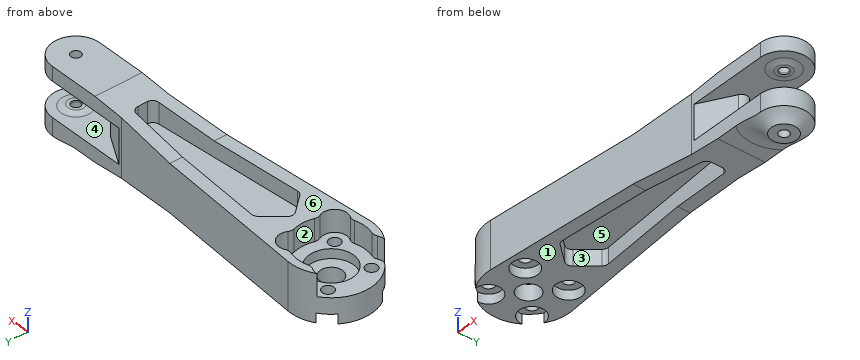
from build123d import *

# Parameters (mm, degrees)
SKETCH2_R               = 13
SKETCH2_R_2             = 7.5
BOSS_EXTRUDE2_DEPTH     = 10
CUT_EXTRUDE1_DEPTH      = 105.791459576
CUT_EXTRUDE1_DEPTH_BACK = 105.791459576
SKETCH5_R               = 1.83
SKETCH5_R_2             = 3.5
CUT_EXTRUDE2_DEPTH      = 106.770979007
HUB_CUTOUT_DEPTH        = 7
SKETCH8_R               = 7
CUT_EXTRUDE4_DEPTH      = 3
CUT_EXTRUDE5_DEPTH      = 105.791459576
CUT_EXTRUDE5_DEPTH_BACK = 105.791459576
SKETCH9_R               = 1.55
CUT_EXTRUDE6_DEPTH      = 5.5
FILLET1_R               = 2
CUT_EXTRUDE7_START      = 2.5
CUT_EXTRUDE7_DEPTH      = 103.291459576
FILLET2_R               = 2
FILLET2_OF_MIRROR1_R    = 2
SKETCH12_R              = 4
SKETCH12_R_2            = 1.55
BOSS_EXTRUDE3_DEPTH     = 4
FILLET3_START           = -14
FILLET3_2_DEPTH         = 4
BOSS_EXTRUDE4_START     = 5.5
SKETCH13_R              = 2.5
SKETCH13_R_2            = 1.5
BOSS_EXTRUDE4_DEPTH     = 0.5
BOSS_EXTRUDE5_START     = -5
SKETCH13_2_R            = 2.5
SKETCH13_2_R_2          = 1.5
BOSS_EXTRUDE5_DEPTH     = 0.5
FILLET4_R               = 5
SKETCH15_R              = 4
CUT_EXTRUDE8_DEPTH      = 3


with BuildPart() as part:
    # Sketch2 → Boss-Extrude2 (new, symmetric)
    with BuildSketch(Plane.XY):
        Circle(SKETCH2_R)
        with BuildLine():
            Line((70, 7.5), (1.025771359, 12.959467316))
            ThreePointArc((1.025771359, 12.959467316), (9.548168088, 8.822272166), (13, 0))
            ThreePointArc((13, 0), (9.548168088, -8.822272166), (1.025771359, -12.959467316))
            Line((1.025771359, -12.959467316), (70, -7.5))
            Line((70, -7.5), (70, 7.5))
        make_face()
        with BuildLine():
            Line((96, 7.5), (70, 7.5))
            Line((70, 7.5), (70, -7.5))
            Line((70, -7.5), (96, -7.5))
            ThreePointArc((96, -7.5), (88.5, 0), (96, 7.5))
        make_face()
        with Locations((96, 0)):
            Circle(SKETCH2_R_2)
        Circle(SKETCH2_R)
    extrude(amount=BOSS_EXTRUDE2_DEPTH, both=True)

    # Sketch4 → Cut-Extrude1 (cut, two sides: drawn at the far end of the back side and taken through both)
    with BuildSketch(Plane(origin=(0, 0, 0), x_dir=(1, 0, 0), z_dir=(0, 1, 0)).offset(-CUT_EXTRUDE1_DEPTH_BACK)):
        Polygon((-13, 7.5), (50, 7.5), (80, 10), (-13, 10), align=None)
        Polygon((-13, -7.5), (50, -7.5), (80, -10), (-13, -10), align=None)
    extrude(amount=CUT_EXTRUDE1_DEPTH + CUT_EXTRUDE1_DEPTH_BACK, mode=Mode.SUBTRACT)

    # Sketch5 → Cut-Extrude2 (cut, through all)
    with BuildSketch(Plane.XY.offset(7.5)):
        with Locations((-6.914797213, 6.914797213)):
            Circle(SKETCH5_R)
        with Locations((6.914797213, 6.914797213)):
            Circle(SKETCH5_R)
        with Locations((6.914797213, -6.914797213)):
            Circle(SKETCH5_R)
        with Locations((-6.914797213, -6.914797213)):
            Circle(SKETCH5_R)
        Circle(SKETCH5_R_2)
    extrude(amount=-CUT_EXTRUDE2_DEPTH, mode=Mode.SUBTRACT)

    # Sketch7 → hub cutout (cut)
    with BuildSketch(Plane.XY.offset(7.5)):
        with BuildLine():
            ThreePointArc((-7.281143007, 10.769631215), (-13, 0), (-7.281143007, -10.769631215))
            ThreePointArc((-7.281143007, -10.769631215), (-6.15529138, -10.711783559), (-5.093815501, -10.332103173))
            ThreePointArc((-5.093815501, -10.332103173), (-4.17580433, -10.057753531), (-3.223255475, -10.161014917))
            ThreePointArc((-3.223255475, -10.161014917), (0, -10.66), (3.223255475, -10.161014917))
            ThreePointArc((3.223255475, -10.161014917), (4.17580433, -10.057753531), (5.093815501, -10.332103173))
            ThreePointArc((5.093815501, -10.332103173), (9.652858062, -9.652858062), (10.332103173, -5.093815501))
            ThreePointArc((10.332103173, -5.093815501), (10.057753531, -4.17580433), (10.161014917, -3.223255475))
            ThreePointArc((10.161014917, -3.223255475), (10.66, 0), (10.161014917, 3.223255475))
            ThreePointArc((10.161014917, 3.223255475), (10.057753531, 4.17580433), (10.332103173, 5.093815501))
            ThreePointArc((10.332103173, 5.093815501), (9.652858062, 9.652858062), (5.093815501, 10.332103173))
            ThreePointArc((5.093815501, 10.332103173), (4.17580433, 10.057753531), (3.223255475, 10.161014917))
            ThreePointArc((3.223255475, 10.161014917), (0, 10.66), (-3.223255475, 10.161014917))
            ThreePointArc((-3.223255475, 10.161014917), (-4.17580433, 10.057753531), (-5.093815501, 10.332103173))
            ThreePointArc((-5.093815501, 10.332103173), (-6.15529138, 10.711783559), (-7.281143007, 10.769631215))
        make_face()
    extrude(amount=-HUB_CUTOUT_DEPTH, mode=Mode.SUBTRACT)

    # Sketch8 → Cut-Extrude4 (cut)
    with BuildSketch(Plane.XY.offset(0.5)):
        Circle(SKETCH8_R)
    extrude(amount=-CUT_EXTRUDE4_DEPTH, mode=Mode.SUBTRACT)

    # Sketch9 → Cut-Extrude5 (cut, two sides: drawn at the far end of the back side and taken through both)
    with BuildSketch(Plane.XY.offset(-CUT_EXTRUDE5_DEPTH_BACK)):
        with Locations((96, 0)):
            Circle(SKETCH9_R)
    extrude(amount=CUT_EXTRUDE5_DEPTH + CUT_EXTRUDE5_DEPTH_BACK, mode=Mode.SUBTRACT)

    # Sketch10 → Cut-Extrude6 (cut, symmetric)
    with BuildSketch(Plane.XY):
        Polygon((84, 0), (62.184725581, 12.595054558), (110.068063566, 12.595054558), (110.068063566, -12.520209035), (62.31436183, -12.520209035), align=None)
    extrude(amount=CUT_EXTRUDE6_DEPTH, both=True, mode=Mode.SUBTRACT)

    # Fillet1
    fillet1_edges = [part.edges().sort_by_distance(p)[0] for p in [
        (84, 0, 0),
    ]]
    fillet(fillet1_edges, radius=FILLET1_R)

    # Sketch11 → Cut-Extrude7 (cut, through all)
    with BuildSketch(Plane.XY.offset(CUT_EXTRUDE7_START)):
        Polygon((13.951045221, 0), (20.381756661, 7.414886386), (70.904413477, 3.415903011), (70.904413477, 0), (70.904413477, -3.415903011), (20.381756661, -7.414886386), align=None)
    cut_extrude7 = extrude(amount=CUT_EXTRUDE7_DEPTH, mode=Mode.SUBTRACT)

    # Fillet2
    fillet2_edges = [part.edges().sort_by_distance(p)[0] for p in [
        (13.951045221, 0, 5),
        (20.381756661, 7.414886386, 5),
        (20.381756661, -7.414886386, 5),
        (70.904413477, -3.415903011, 5.871017228),
        (70.904413477, 3.415903011, 5.871017228),
    ]]
    fillet(fillet2_edges, radius=FILLET2_R)

    # Mirror1: Cut-Extrude7 across plane
    add(cut_extrude7.mirror(Plane.XY), mode=Mode.SUBTRACT)

    # Fillet2 of Mirror1
    fillet2_of_mirror1_edges = [part.edges().sort_by_distance(p)[0] for p in [
        (13.951045221, 0, -5),
        (20.381756661, 7.414886386, -5),
        (20.381756661, -7.414886386, -5),
        (70.904413477, -3.415903011, -5.871017228),
        (70.904413477, 3.415903011, -5.871017228),
    ]]
    fillet(fillet2_of_mirror1_edges, radius=FILLET2_OF_MIRROR1_R)

    # Sketch12 → Boss-Extrude3 (add)
    with BuildSketch(Plane(origin=(0, 0, -10), x_dir=(-1, 0, 0), z_dir=(0, 0, -1))):
        with Locations(Location((-96, 0, 0), (0, 0, 180))):
            Circle(SKETCH12_R)
        with Locations(Location((-96, 0, 0), (0, 0, 180))):
            Circle(SKETCH12_R_2, mode=Mode.SUBTRACT)
    extrude(amount=BOSS_EXTRUDE3_DEPTH)

    # Fillet3: read off the stored shape, not the designer's step
    # Fillet3 outline → Fillet3 (revolve)
    with BuildSketch(Plane(origin=(96, 0, 0), x_dir=(1, 0, 0), z_dir=(0, -1, 0))):
        with BuildLine():
            ThreePointArc((4, -14), (7.527864045, -11.05572809), (12, -10))
            Line((12, -10), (4, -10))
            Line((4, -10), (4, -14))
        make_face()
    revolve(axis=Axis((96, 0, 0), (0, 0, 1)))

    # Fillet3 2 outline → Fillet3 2 (cut)
    with BuildSketch(Plane.XY.offset(FILLET3_START)):
        with BuildLine():
            ThreePointArc((96, 7.5), (103.5, 0), (96, -7.5))
            Line((96, -7.5), (85, -7.5))
            Line((85, -7.5), (85, -13))
            Line((85, -13), (109, -13))
            Line((109, -13), (109, 13))
            Line((109, 13), (85, 13))
            Line((85, 13), (85, 7.5))
            Line((85, 7.5), (96, 7.5))
        make_face()
    extrude(amount=FILLET3_2_DEPTH, mode=Mode.SUBTRACT)

    # Sketch13 → Boss-Extrude4 (add)
    with BuildSketch(Plane.XY.offset(BOSS_EXTRUDE4_START)):
        with Locations((96, 0)):
            Circle(SKETCH13_R)
        with Locations((96, 0)):
            Circle(SKETCH13_R_2, mode=Mode.SUBTRACT)
    extrude(amount=-BOSS_EXTRUDE4_DEPTH)

    # Sketch13<2> → Boss-Extrude5 (add)
    with BuildSketch(Plane.XY.offset(BOSS_EXTRUDE5_START)):
        with Locations((96, 0)):
            Circle(SKETCH13_2_R)
        with Locations((96, 0)):
            Circle(SKETCH13_2_R_2, mode=Mode.SUBTRACT)
    extrude(amount=-BOSS_EXTRUDE5_DEPTH)

    # Fillet4
    # the kernel refuses this fillet: 5 mm, written as the material it adds along each edge
    with BuildSketch(Plane(origin=(96, 0, 5.5), x_dir=(1, 0, 0), z_dir=(0, -1, 0))) as fillet4_piece_1:
        with BuildLine():
            CenterArc((4.679449472, -5), FILLET4_R, 90, 25.841932763)
            Line((2.5, -0.5), (2.456411011, -0.41))
            ThreePointArc((2.456411011, -0.41), (2.4, -0.25), (2.4, 0))
            Line((2.4, 0), (2.5, 0.1))
            Line((2.5, 0.1), (4.679449472, 0.1))
            Line((4.679449472, 0.1), (4.679449472, 0))
        make_face()
    revolve(axis=Axis((96, 0, 5.5), (0, 0, 1)))
    with BuildSketch(Plane(origin=(96, 0, -5.5), x_dir=(1, 0, 0), z_dir=(0, -1, 0))) as fillet4_piece_2:
        with BuildLine():
            CenterArc((4.679449472, 5), FILLET4_R, 244.158067237, 25.841932763)
            Line((2.5, 0.5), (2.456411011, 0.41))
            ThreePointArc((2.456411011, 0.41), (2.4, 0.25), (2.4, 0))
            Line((2.4, 0), (2.5, -0.1))
            Line((2.5, -0.1), (4.679449472, -0.1))
            Line((4.679449472, -0.1), (4.679449472, 0))
        make_face()
    revolve(axis=Axis((96, 0, -5.5), (0, 0, 1)))

    # Sketch15 → Cut-Extrude8 (cut)
    with BuildSketch(Plane(origin=(0, 0, -7.5), x_dir=(-1, 0, 0), z_dir=(0, 0, -1))):
        with Locations((6.914797213, -6.914797213)):
            Circle(SKETCH15_R)
        with Locations((-6.914797213, -6.914797213)):
            Circle(SKETCH15_R)
        with Locations((6.914797213, 6.914797213)):
            Circle(SKETCH15_R)
        with Locations((-6.914797213, 6.914797213)):
            Circle(SKETCH15_R)
    extrude(amount=-CUT_EXTRUDE8_DEPTH, mode=Mode.SUBTRACT)


solid = part.part
CAD build for the part. Positions are in the model's coordinates, mm. Face numbers are marked on the shaded views. A direction names the side the tool comes from. Round coordinates to 2 decimals unless told otherwise and drop trailing zeros. Loops run counter-clockwise (first coordinate to the right, second up) from the corner with the lowest first, then second, coordinate; pieces in that order, holes last.
(1) Cut at C-C (x = 38.5). Give the cut face in (y, z).
(2) Two-plate mould, pull along X, no slides. Class the marked faces 1, 2 and 3: +X half, -X half, draft (parallel to the pull), parting line (faces both ways), or undercut.
(3) Cut at B-B (y = 0). State how many separate pieces and enclosed holes the cut face has, plus the area to 3 significant figures.
(4) Wall check: line 1 along Y through (x, z) = (0, -0.85); line 2 along Y through (x, z) = (96, 8); line 3 along X through (y, z) = (-0.5, -4.25). Give the ranges that are in metal, low to high.
(5) Which spindle directions (+Z, -Z, +X, -X, +Y, -Y) get a long thin tool onto all of the face, cutting with end or side? Do the marked faces 4, 5 and 6. Say none if no direction does.
(6) Cut at A-A (x = 0). Give the cut face in (y, z), plus the area to 3 significant figures.
(7) Cut at D-D (x = 51.5). Give the cut face in (y, z) (3 decimals), plus the area to 3 significant figures.
(8) Drop flat-ended pins along their axis: pin 1 (12 mm diameter, centred on x = 26.5, z = -8, fed in from -Y); pin 2 (8 mm diameter, centred on x = 24.5, y = 4, fed in from +Z); pin 3 (2.5 mm diameter, centred on x = 96.5, y = -0.5, fed in from +Z); pin 4 (0.9 mm diameter, centred on y = 0.5, z = 7.5, fed in from -X). Give the stop position or say it passes through.
Findings below:
1. outline: (-9.99, -7.5) - (-5.98, -7.5) - (-5.98, -2.5) - (5.98, -2.5) - (5.98, -7.5) - (9.99, -7.5) - (9.99, 7.5) - (5.98, 7.5) - (5.98, 2.5) - (-5.98, 2.5) - (-5.98, 7.5) - (-9.99, 7.5) - close
2. face 1: draft
2. face 2: -X half
2. face 3: undercut
3. separate pieces: 4
3. enclosed holes: 0
3. area: 874 mm2
4. line 1: y = -13 to -7, 7 to 13
4. line 2: y = -7.5 to -1.55, 1.55 to 7.5
4. line 3: x = -12.99 to -3.46, 3.46 to 14.66, 70.9 to 81.94
5. face 4: none
5. face 5: -Z
5. face 6: +Z, -X, +Y, -Y
6. outline: (-13, -7.5) - (-3.5, -7.5) - (-3.5, -2.5) - (-7, -2.5) - (-7, 0.5) - (-10.66, 0.5) - (-10.66, 7.5) - (-13, 7.5) - close; (3.5, -7.5) - (13, -7.5) - (13, 7.5) - (10.66, 7.5) - (10.66, 0.5) - (7, 0.5) - (7, -2.5) - (3.5, -2.5) - close
6. area: 164 mm2
7. outline: (-8.964, -7.625) - (-4.952, -7.625) - (-4.952, -2.5) - (4.952, -2.5) - (4.952, -7.625) - (8.964, -7.625) - (8.964, 7.625) - (4.952, 7.625) - (4.952, 2.5) - (-4.952, 2.5) - (-4.952, 7.625) - (-8.964, 7.625) - close
7. area: 172 mm2
8. pin 1: stops at y = -11.42
8. pin 2: stops at z = 7.5
8. pin 3: stops at z = 10
8. pin 4: stops at x = 10.62
